Source: CAD feature listing. Evaluate the final solid. Frame: model axes, mm. Give positions to 0.01 mm unless a question says otherwise; leave off trailing zeros. Loops run counter-clockwise (first coordinate to the right, second up) from the corner with the lowest first, then second, coordinate; pieces in that order, holes last. Notation, with made-up numbers: M 26,45 L 59,45 A28 ccw 59,80 Z; hole C 74.25,19 d1. An arc over 180 degrees is marked long. Answer in a Markdown table with one row per item.
```python
from build123d import *

# Parameters (mm, degrees)
F0_W     = 341.3125
F0_H     = 598.5927322
F0_R     = 2.15265
F0_W_2   = 273.05
F0_H_2   = 530.3302322
F1_DEPTH = 1.5875
F2_R     = 4.7625
F3_W     = 25.4
F3_H     = 7.14375
F4_DEPTH = 1.5875
F5_SIZE  = 1.5875


with BuildPart() as f1:
    # F0 (on Top) → F1 (new body)
    with BuildSketch(Plane.XY):
        Rectangle(F0_W, F0_H)
        with Locations((-140.49375, -269.1338661)):
            Circle(F0_R, mode=Mode.SUBTRACT)
        with Locations((140.49375, -269.1338661)):
            Circle(F0_R, mode=Mode.SUBTRACT)
        with Locations((-140.49375, 269.1338661)):
            Circle(F0_R, mode=Mode.SUBTRACT)
        Rectangle(F0_W_2, F0_H_2, mode=Mode.SUBTRACT)
        with Locations((140.49375, 269.1338661)):
            Circle(F0_R, mode=Mode.SUBTRACT)
    extrude(amount=F1_DEPTH)

    # F2
    f2_edges = [f1.edges().sort_by_distance(p)[0] for p in [
        (-170.65625, 299.296366, 0.79375),
        (170.65625, 299.296366, 0.79375),
        (170.65625, -299.296366, 0.79375),
        (-170.65625, -299.296366, 0.79375),
    ]]
    fillet(f2_edges, radius=F2_R)

    # F3 (on face) → F4 (cut, through all)
    with BuildSketch(Plane.XY.offset(1.5875)):
        with Locations((0, -268.7369911)):
            Rectangle(F3_W, F3_H)
    extrude(amount=-F4_DEPTH, mode=Mode.SUBTRACT)

    # F5
    f5_edges = [f1.edges().sort_by_distance(p)[0] for p in [
        (12.7, -265.165116, 0.79375),
        (-12.7, -265.165116, 0.79375),
    ]]
    chamfer(f5_edges, length=F5_SIZE)


solid = f1.part
```
1) Section C-C, the plane z = 0.55. Return loops of the section in (x, y) (1 decimal).
Reply:
| item | result |
|---|---|
| outline | M -170.7,-294.5 A4.8 ccw -165.9,-299.3 L 165.9,-299.3 A4.8 ccw 170.7,-294.5 L 170.7,294.5 A4.8 ccw 165.9,299.3 L -165.9,299.3 A4.8 ccw -170.7,294.5 Z; hole C -140.5,-269.1 d4.3; hole C -140.5,269.1 d4.3; hole M -136.5,-265.2 L -14.3,-265.2 L -12.7,-266.8 L -12.7,-272.3 L 12.7,-272.3 L 12.7,-266.8 L 14.3,-265.2 L 136.5,-265.2 L 136.5,265.2 L -136.5,265.2 Z; hole C 140.5,-269.1 d4.3; hole C 140.5,269.1 d4.3 |
2) Section A-A, the plane y = 103. Return loops of the section in (x, z) (1 decimal), then the cut area to 3 significant figures.
Reply:
| item | result |
|---|---|
| outline | M -170.7,0 L -136.5,0 L -136.5,1.6 L -170.7,1.6 Z; M 136.5,0 L 170.7,0 L 170.7,1.6 L 136.5,1.6 Z |
| area | 108 mm² |
3) Pin query (flat end, axial travel): pin 1 Ø5 at (x, y) = (-140.49, -269.13) entering from -Z. Return the tip coordinate at first contact, or that it passes through.
Reply:
| item | result |
|---|---|
| pin 1 | stops at z = 0 |
4) Section B-B, the plane x = 47. Return loops of the section in (y, z).
Reply:
| item | result |
|---|---|
| outline | M -299.3,0 L -265.17,0 L -265.17,1.59 L -299.3,1.59 Z; M 265.17,0 L 299.3,0 L 299.3,1.59 L 265.17,1.59 Z |
5) Material intervals for L1, parallel to Y at x = 140, z = 0.45; L2, parallel to X at y = -0.5, z = 0.2 (3 decimals); L3, parallel to Y at x = -95.5, z = 0.6, sorted ascending.
Reply:
| item | result |
|---|---|
| L1 | y = -299.3 to -271.23, -267.04 to 267.04, 271.23 to 299.3 |
| L2 | x = -170.656 to -136.525, 136.525 to 170.656 |
| L3 | y = -299.3 to -265.17, 265.17 to 299.3 |
